```python
from build123d import *

# Parameters (mm, degrees)
AUFSATZ_LINEAR_AUSTRAGEN1_DEPTH = 4
SKIZZE2_W                       = 19.8
SKIZZE2_H                       = 3.7
SCHNITT_LINEAR_AUSTRAGEN1_DEPTH = 4
SPIEGELN2_COPY_1_SKETCH_W       = 19.8
SPIEGELN2_COPY_1_SKETCH_H       = 3.7
SPIEGELN2_COPY_1_DEPTH          = 4
SCHNITT_LINEAR_AUSTRAGEN2_DEPTH = 4
LINEARES_MUSTER1_COUNT          = 8
LINEARES_MUSTER1_PITCH          = 20
LINEARES_MUSTER1_COPY_1_DEPTH   = 4
LINEARES_MUSTER1_COPY_2_DEPTH   = 4
LINEARES_MUSTER1_COPY_3_DEPTH   = 4
LINEARES_MUSTER1_COPY_4_DEPTH   = 4
LINEARES_MUSTER1_COPY_5_DEPTH   = 4
LINEARES_MUSTER1_COPY_6_DEPTH   = 4
LINEARES_MUSTER1_COPY_7_DEPTH   = 4


with BuildPart() as part:
    # Skizze1 → Aufsatz-Linear austragen1 (new body)
    with BuildSketch(Plane.XY):
        Polygon((35.01037691, 0), (0, 50), (0, 120), (35.01037691, 170), (280, 170), (280, 0), align=None)
    extrude(amount=AUFSATZ_LINEAR_AUSTRAGEN1_DEPTH)

    # Skizze2 → Schnitt-Linear austragen1 (cut)
    with BuildSketch(Plane.XY.offset(4)):
        with Locations((28.7, 155.75)):
            Rectangle(SKIZZE2_W, SKIZZE2_H)
        with Locations((28.7, 133.25)):
            Rectangle(SKIZZE2_W, SKIZZE2_H)
    schnitt_linear_austragen1 = extrude(amount=-SCHNITT_LINEAR_AUSTRAGEN1_DEPTH, mode=Mode.SUBTRACT)

    # Spiegeln1: Schnitt-Linear austragen1 across plane
    add(schnitt_linear_austragen1.mirror(Plane.ZX.offset(85)), mode=Mode.SUBTRACT)

    # Spiegeln2: Schnitt-Linear austragen1 across plane
    add(schnitt_linear_austragen1.mirror(Plane.ZY.offset(-140)), mode=Mode.SUBTRACT)

    # Spiegeln2 copy 1 sketch → Spiegeln2 copy 1 (cut)
    with BuildSketch(Plane(origin=(280, 170, 4), x_dir=(-1, 0, 0), z_dir=(0, 0, 1))):
        with Locations((28.7, 155.75)):
            Rectangle(SPIEGELN2_COPY_1_SKETCH_W, SPIEGELN2_COPY_1_SKETCH_H)
        with Locations((28.7, 133.25)):
            Rectangle(SPIEGELN2_COPY_1_SKETCH_W, SPIEGELN2_COPY_1_SKETCH_H)
    extrude(amount=-SPIEGELN2_COPY_1_DEPTH, mode=Mode.SUBTRACT)

    # Skizze4 → Schnitt-Linear austragen2 (cut)
    with BuildSketch(Plane.XY.offset(4)):
        with BuildLine():
            Line((69.37540934, 85), (74.37540934, 85))
            Line((74.37540934, 85), (74.37540934, 125))
            ThreePointArc((74.37540934, 125), (71.87540934, 127.5), (69.37540934, 125))
            Line((69.37540934, 125), (69.37540934, 85))
        make_face()
    schnitt_linear_austragen2 = extrude(amount=-SCHNITT_LINEAR_AUSTRAGEN2_DEPTH, mode=Mode.SUBTRACT)

    # Spiegeln3: Schnitt-Linear austragen2 across plane
    add(schnitt_linear_austragen2.mirror(Plane.ZX.offset(85)), mode=Mode.SUBTRACT)

    # Lineares Muster1: Schnitt-Linear austragen2 ×8
    with Locations(*[(i * LINEARES_MUSTER1_PITCH, 0, 0) for i in range(1, LINEARES_MUSTER1_COUNT)]):
        add(schnitt_linear_austragen2, mode=Mode.SUBTRACT)

    # Lineares Muster1 copy 1 sketch → Lineares Muster1 copy 1 (cut)
    with BuildSketch(Plane(origin=(20, 170, 4), x_dir=(1, 0, 0), z_dir=(0, 0, 1))):
        with BuildLine():
            Line((69.37540934, -85), (74.37540934, -85))
            Line((74.37540934, -85), (74.37540934, -125))
            ThreePointArc((74.37540934, -125), (71.87540934, -127.5), (69.37540934, -125))
            Line((69.37540934, -125), (69.37540934, -85))
        make_face()
    extrude(amount=-LINEARES_MUSTER1_COPY_1_DEPTH, mode=Mode.SUBTRACT)

    # Lineares Muster1 copy 2 sketch → Lineares Muster1 copy 2 (cut)
    with BuildSketch(Plane(origin=(40, 170, 4), x_dir=(1, 0, 0), z_dir=(0, 0, 1))):
        with BuildLine():
            Line((69.37540934, -85), (74.37540934, -85))
            Line((74.37540934, -85), (74.37540934, -125))
            ThreePointArc((74.37540934, -125), (71.87540934, -127.5), (69.37540934, -125))
            Line((69.37540934, -125), (69.37540934, -85))
        make_face()
    extrude(amount=-LINEARES_MUSTER1_COPY_2_DEPTH, mode=Mode.SUBTRACT)

    # Lineares Muster1 copy 3 sketch → Lineares Muster1 copy 3 (cut)
    with BuildSketch(Plane(origin=(60, 170, 4), x_dir=(1, 0, 0), z_dir=(0, 0, 1))):
        with BuildLine():
            Line((69.37540934, -85), (74.37540934, -85))
            Line((74.37540934, -85), (74.37540934, -125))
            ThreePointArc((74.37540934, -125), (71.87540934, -127.5), (69.37540934, -125))
            Line((69.37540934, -125), (69.37540934, -85))
        make_face()
    extrude(amount=-LINEARES_MUSTER1_COPY_3_DEPTH, mode=Mode.SUBTRACT)

    # Lineares Muster1 copy 4 sketch → Lineares Muster1 copy 4 (cut)
    with BuildSketch(Plane(origin=(80, 170, 4), x_dir=(1, 0, 0), z_dir=(0, 0, 1))):
        with BuildLine():
            Line((69.37540934, -85), (74.37540934, -85))
            Line((74.37540934, -85), (74.37540934, -125))
            ThreePointArc((74.37540934, -125), (71.87540934, -127.5), (69.37540934, -125))
            Line((69.37540934, -125), (69.37540934, -85))
        make_face()
    extrude(amount=-LINEARES_MUSTER1_COPY_4_DEPTH, mode=Mode.SUBTRACT)

    # Lineares Muster1 copy 5 sketch → Lineares Muster1 copy 5 (cut)
    with BuildSketch(Plane(origin=(100, 170, 4), x_dir=(1, 0, 0), z_dir=(0, 0, 1))):
        with BuildLine():
            Line((69.37540934, -85), (74.37540934, -85))
            Line((74.37540934, -85), (74.37540934, -125))
            ThreePointArc((74.37540934, -125), (71.87540934, -127.5), (69.37540934, -125))
            Line((69.37540934, -125), (69.37540934, -85))
        make_face()
    extrude(amount=-LINEARES_MUSTER1_COPY_5_DEPTH, mode=Mode.SUBTRACT)

    # Lineares Muster1 copy 6 sketch → Lineares Muster1 copy 6 (cut)
    with BuildSketch(Plane(origin=(120, 170, 4), x_dir=(1, 0, 0), z_dir=(0, 0, 1))):
        with BuildLine():
            Line((69.37540934, -85), (74.37540934, -85))
            Line((74.37540934, -85), (74.37540934, -125))
            ThreePointArc((74.37540934, -125), (71.87540934, -127.5), (69.37540934, -125))
            Line((69.37540934, -125), (69.37540934, -85))
        make_face()
    extrude(amount=-LINEARES_MUSTER1_COPY_6_DEPTH, mode=Mode.SUBTRACT)

    # Lineares Muster1 copy 7 sketch → Lineares Muster1 copy 7 (cut)
    with BuildSketch(Plane(origin=(140, 170, 4), x_dir=(1, 0, 0), z_dir=(0, 0, 1))):
        with BuildLine():
            Line((69.37540934, -85), (74.37540934, -85))
            Line((74.37540934, -85), (74.37540934, -125))
            ThreePointArc((74.37540934, -125), (71.87540934, -127.5), (69.37540934, -125))
            Line((69.37540934, -125), (69.37540934, -85))
        make_face()
    extrude(amount=-LINEARES_MUSTER1_COPY_7_DEPTH, mode=Mode.SUBTRACT)


solid = part.part
```
Model file for the job. Use its own axes, mm. Coordinates: 2 decimals unless noted, no trailing zeros. Write each loop counter-clockwise with the first axis right and the second up, starting at its lowest first coordinate (ties: lowest second). Pieces come first, ordered by that corner, then holes. Notation, with made-up numbers: (-30, 65.5) - (2, 65.5) arc R21 cw to (2, 87.5) - close; hole circle Ø3 at (-22.75, -34.75). An arc over 180 degrees is marked (long way). Use a Markdown table: item, result. Add a question column.
Item 1: Band-saw the part on C-C, the plane y = 22.5. Write the cut outline in (x, z), and give its area (3 significant figures).
Item 2: Band-saw the part on D-D, the plane y = 142.5. Write the cut outline in (x, z).
Item 3: Drop flat-ended pins along their axis: pin 1 (8 mm diameter, centred on x = 149, y = 60.5, fed in from -Z); pin 2 (1.1 mm diameter, centred on y = 15, z = 2.5, fed in from -X). Give the stop position or say it passes through.
Item 4: Band-saw the part on A-A, the plane y = 110.5. Give the number of separate pieces and of enclosed holes in the cut face, and give its area (3 significant figures).
Item 5: Drill centre lines: line 1 along Y through (x, z) = (154, 0.75); line 2 along X through (y, z) = (8.5, 2.7); line 3 along X through (y, z) = (23.5, 0.4). Where is each one in solid material? Low to high.
A:
| question | item | result |
|---|---|---|
| 1 | outline | (19.26, 0) - (280, 0) - (280, 4) - (19.26, 4) - close |
| 1 | area | 1,040 mm² |
| 2 | outline | (15.75, 0) - (280, 0) - (280, 4) - (15.75, 4) - close |
| 3 | pin 1 | stops at z = 0 |
| 3 | pin 2 | stops at x = 38.6 |
| 4 | separate pieces | 9 |
| 4 | enclosed holes | 0 |
| 4 | area | 960 mm² |
| 5 | line 1 | y = 0 to 43.68, 126.32 to 170 |
| 5 | line 2 | x = 29.06 to 280 |
| 5 | line 3 | x = 18.56 to 280 |
